Build history of the part. All positions in model axes, mm. Face numbers are marked on the shaded views. A direction names the side the tool comes from. Coordinates: 2 decimals unless noted, no trailing zeros. Write each loop counter-clockwise with the first axis right and the second up, starting at its lowest first coordinate (ties: lowest second). Pieces come first, ordered by that corner, then holes.
from build123d import *

# Parameters (mm, degrees)
BOSS_EXTRU_1_DEPTH = 5


with BuildPart() as part:
    # Esquisse1 → Révolution1 (revolve)
    with BuildSketch(Plane(origin=(0, 0, 0), x_dir=(1, 0, 0), z_dir=(0, 1, 0))):
        Polygon((-2.5, 0), (-6.1, 0), (-6.1, 2), (-4.1, 2), (-4.1, 7), (-2.5, 7), align=None)
    revolve(axis=Axis((0, 0, -7.597402597), (0, 0, 1)))

    # Esquisse2 → Boss.-Extru.1 (add)
    with BuildSketch(Plane(origin=(0, 0, -7), x_dir=(-1, 0, 0), z_dir=(0, 0, -1))):
        with BuildLine():
            Line((-2.899137803, 2.899137803), (-1.767766953, 1.767766953))
            ThreePointArc((-1.767766953, 1.767766953), (-2.5, 0), (-1.767766953, -1.767766953))
            Line((-1.767766953, -1.767766953), (-2.899137803, -2.899137803))
            ThreePointArc((-2.899137803, -2.899137803), (-4.1, 0), (-2.899137803, 2.899137803))
        make_face()
    extrude(amount=BOSS_EXTRU_1_DEPTH)


solid = part.part
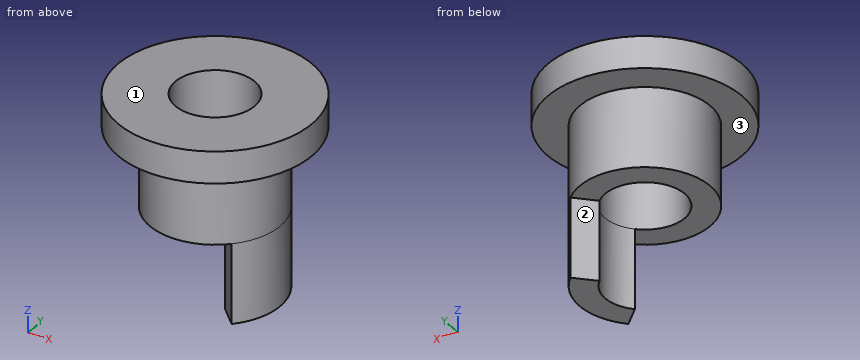
(1) Probe L1, parallel to Y at x = 0, z = -2.5; L2, parallel to Y at x = 0, z = -1.75. List the from-to ranges inside material, lowest first.
(2) Slice it at C-C, the plane y = 2.25. List the corners of the cut face in (x, z), and give its area (3 significant figures).
(3) Flat gauge pins, fed straight in: P1, Ø2, axis at x = 4.5, y = 4.5, coming from the -Z side; P2, Ø2, axis at y = 0.5, z = -7.5, coming from the -X side; P3, Ø4, axis at y = -4, z = -1.5, coming from the -X side. Where does each tip first touch, or does it go through?
(4) 3-axis set-ups, long thin cutter, end or side, ignore diameter. For the marked faces 1, 2 and 3: which of +Z, -Z, +X, -X, +Y, -Y reach the whole face in a straight line?
(5) Slice it at A-A, the plane y = 0. List the corners of the cut face in (x, z), and give its area (3 significant figures).
(6) Slice it at B-B, the plane x = 0. List the corners of the cut face in (y, z).
(7) Slice it at D-D, the plane x = -3. List the corners of the cut face in (y, z).
Results:
1. L1: y = -4.1 to -2.5, 2.5 to 4.1
1. L2: y = -6.1 to -2.5, 2.5 to 6.1
2. outline: (-5.67, -2) - (-3.43, -2) - (-3.43, -7) - (-1.09, -7) - (-1.09, 0) - (-5.67, 0) - close; (1.09, -7) - (2.25, -7) - (2.25, -12) - (3.43, -12) - (3.43, -2) - (5.67, -2) - (5.67, 0) - (1.09, 0) - close
2. area: 47.6 mm2
3. P1: stops at z = -2
3. P2: stops at x = -4.1
3. P3: stops at x = -5.76
4. face 1: +Z, +X, -X, +Y, -Y
4. face 2: -Z, -X, +Y
4. face 3: -Z
5. outline: (-6.1, -2) - (-4.1, -2) - (-4.1, -7) - (-2.5, -7) - (-2.5, 0) - (-6.1, 0) - close; (2.5, -12) - (4.1, -12) - (4.1, -2) - (6.1, -2) - (6.1, 0) - (2.5, 0) - close
5. area: 38.4 mm2
6. outline: (-6.1, -2) - (-4.1, -2) - (-4.1, -7) - (-2.5, -7) - (-2.5, 0) - (-6.1, 0) - close; (2.5, -7) - (4.1, -7) - (4.1, -2) - (6.1, -2) - (6.1, 0) - (2.5, 0) - close
7. outline: (-5.31, -2) - (-2.79, -2) - (-2.79, -7) - (2.79, -7) - (2.79, -2) - (5.31, -2) - (5.31, 0) - (-5.31, 0) - close
